Verification items for the finished model (mm, model axes). Give positions to 0.01 mm unless a question says otherwise; leave off trailing zeros. Write each loop counter-clockwise with the first axis right and the second up, starting at its lowest first coordinate (ties: lowest second). Pieces come first, ordered by that corner, then holes. Notation, with made-up numbers: (23.25, -23.75) -> (44.25, -23.75) arc R14 ccw to (44.25, -10.75) -> close; hole circle Ø3 at (-36, 50). An arc over 180 degrees is marked (long way). Use one line per item in the form item = value. Start each with the question number.
(1) Section check B-B, the plane y = 7.5. Record the cut outline in (x, z), plus the area to 3 significant figures.
(2) Depth check by flat-ended pin: pin 1 Ø6 at (x, y) = (-152.5, 8.5) entering from -Z; pin 2 Ø1.5 at (x, z) = (-151, -110.5) entering from +Y; pin 3 Ø1.5 at (x, y) = (-48.5, 6.5) entering from -Z; pin 4 Ø4 at (x, z) = (-111, 24.5) entering from -Y. Enter the tip coordinate at first touch or a pass-through.
(3) Section check A-A, the plane x = -59.5. Record the cut outline in (y, z).
(4) Scan lines: L1, parallel to Y at x = -171.5, z = -28; L2, parallel to Z at x = -76.5, y = 5.5; L3, parallel to Z at x = -148, y = 2.25. Record each from-to range of solid material in increasing order.
(5) Section check C-C, the plane x = -132. Record the cut outline in (y, z), plus the area to 3 significant figures.
(6) Section check D-D, the plane x = -111.5. Record the cut outline in (y, z).
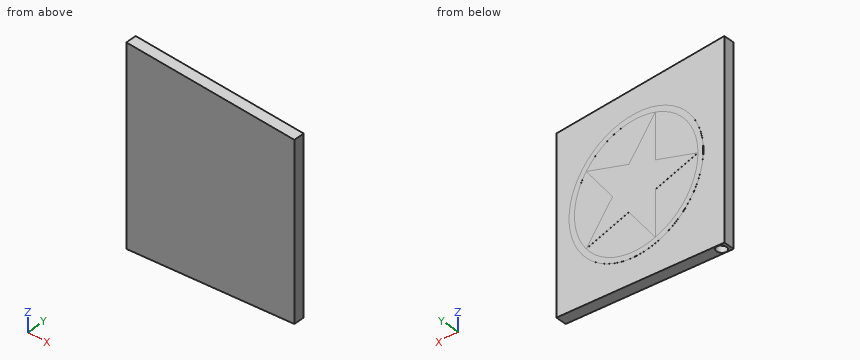
from build123d import *

# Parameters (mm, degrees)
BOSS_EXTRUDE1_DEPTH = 10
SKETCH3_R           = 4.62
CUT_EXTRUDE3_DEPTH  = 6
SKETCH4_R           = 62.5
SKETCH4_R_2         = 57.5
BOSS_EXTRUDE2_DEPTH = 0.05


with BuildPart() as part:
    # Sketch1 → Boss-Extrude1 (new body)
    with BuildSketch(Plane(origin=(0, 0, 0), x_dir=(1, 0, 0), z_dir=(0, 1, 0))):
        Polygon((-180.91295082, 131.617868852), (-180.91295082, -48.802131148), (-24.57295082, -39.020839837), (-24.57295082, 121.836577542), align=None)
    extrude(amount=BOSS_EXTRUDE1_DEPTH)

    # Sketch3 → Cut-Extrude3 (cut)
    with BuildSketch(Plane(origin=(7.497080179, 0, -119.83014083), x_dir=(-0.9980485856506585, 0, -0.062442138662287344), z_dir=(0.062442138662287344, 0, -0.9980485856506585))):
        with Locations((181.778415909, 4.88)):
            Circle(SKETCH3_R)
    extrude(amount=-CUT_EXTRUDE3_DEPTH, mode=Mode.SUBTRACT)

    # Sketch4 → Boss-Extrude2 (add)
    # profile 1 of 2: a face of its own
    with BuildSketch(Plane(origin=(0, 10, 0), x_dir=(1, 0, 0), z_dir=(0, 1, 0))):
        with Locations(Location((-98.92295082, 41.407868852, 0), (0, 0, 90))):
            Circle(SKETCH4_R)
        with Locations(Location((-98.92295082, 41.407868852, 0), (0, 0, 270))):
            Circle(SKETCH4_R_2, mode=Mode.SUBTRACT)
    # profile 2 of 2: a face of its own
    with BuildSketch(Plane(origin=(0, 10, 0), x_dir=(1, 0, 0), z_dir=(0, 1, 0))):
        Polygon((-76.965923859, 41.406760564), (-52.409995832, 75.197921831), (-92.136802298, 62.289899942), (-116.685907341, 96.086018397), (-116.685907341, 54.314782109), (-156.414016678, 41.410770734), (-116.687210213, 28.502748845), (-116.691427048, -13.26848723), (-92.138910388, 20.525152803), (-52.413407199, 7.613120531), align=None)
    extrude(amount=BOSS_EXTRUDE2_DEPTH)


solid = part.part
Completed:
q1.outline = (-180.91, -131.62) -> (-177.72, -131.42) -> (-178.1, -125.43) -> (-170.5, -124.95) -> (-170.13, -130.94) -> (-24.57, -121.84) -> (-24.57, 39.02) -> (-180.91, 48.8) -> close
q1.area = 26,600 mm²
q2.pin_1 = -130.03
q2.pin_2 = 10
q2.pin_3 = -123.38
q2.pin_4 = 0
q3.outline = (0, -124.02) -> (10, -124.02) -> (10, -89.91) -> (10.05, -89.91) -> (10.05, -83.27) -> (10, -83.27) -> (10, -72.89) -> (10.05, -72.89) -> (10.05, -65.44) -> (10, -65.44) -> (10, -17.37) -> (10.05, -17.37) -> (10.05, -9.92) -> (10, -9.92) -> (10, 0.45) -> (10.05, 0.45) -> (10.05, 7.09) -> (10, 7.09) -> (10, 41.21) -> (0, 41.21) -> close
q4.L1 = 0 to 10
q4.L2 = -125.09 to 42.27
q4.L3 = -129.56 to 46.74
q5.outline = (0, -128.56) -> (10, -128.56) -> (10, -94.44) -> (10.05, -94.44) -> (10.05, -88.44) -> (10, -88.44) -> (10, -49.34) -> (10.05, -49.34) -> (10.05, -33.48) -> (10, -33.48) -> (10, 5.63) -> (10.05, 5.63) -> (10.05, 11.62) -> (10, 11.62) -> (10, 45.74) -> (0, 45.74) -> close
q5.area = 1,740 mm²
q6.outline = (0, -127.28) -> (10, -127.28) -> (10, -102.63) -> (10.05, -102.63) -> (10.05, -97.52) -> (10, -97.52) -> (10, -88.95) -> (10.05, -88.95) -> (10.05, 6.12) -> (10, 6.12) -> (10, 14.7) -> (10.05, 14.7) -> (10.05, 19.81) -> (10, 19.81) -> (10, 44.46) -> (0, 44.46) -> close
